Could you check a few things on this model? Use its own coordinates, in mm. Face numbers are marked on the shaded views. Coordinates: 2 decimals unless noted, no trailing zeros. Write each loop counter-clockwise with the first axis right and the second up, starting at its lowest first coordinate (ties: lowest second). Pieces come first, ordered by that corner, then holes. Notation, with made-up numbers: (52, 32) - (74, 32) arc R14 ccw to (74, 54) - close; hole circle Ø1 at (-24.75, 30.25). An arc over 180 degrees is marked (long way). Write item = value, one per line. Start each with the question number.
Autodesk Fusion 360 part; units mm, degrees
sketch "base Sketch" plane through (0, 0, 0) normal (0, 1, 0) x (1, 0, 0)
  line L0 (12.9, -8.5) -> (-12.9, -8.5)
  line L1 (-12.9, -8.5) -> (-12.9, 8.5)
  line L2 (-12.9, 8.5) -> (12.9, 8.5)
  line L3 (12.9, 8.5) -> (12.9, -8.5)
  line L4 (12.9, -8.5) -> (-12.9, 8.5) construction
  line L5 (-12.9, -8.5) -> (12.9, 8.5) construction
  circle A0 centre (5.625, 0) radius 2.775
  circle A1 centre (5.625, 0) radius 1.875
  circle A2 centre (-6.4, -0.0017) radius 2.0246 construction
  line L6 (-6.3962, -4.2517) -> (-2.7175, -2.1234)
  line L7 (-2.7175, -2.1234) -> (-2.7213, 2.1266)
  line L8 (-2.7213, 2.1266) -> (-6.4038, 4.2483)
  line L9 (-6.4038, 4.2483) -> (-10.0825, 2.12)
  line L10 (-10.0825, 2.12) -> (-10.0787, -2.13)
  line L11 (-10.0787, -2.13) -> (-6.3962, -4.2517)
  line L12 (-6.4027, 2.9781) -> (-8.9819, 1.4859)
  line L13 (-8.9819, 1.4859) -> (-8.9793, -1.4939)
  line L14 (-8.9793, -1.4939) -> (-6.3973, -2.9815)
  line L15 (-6.3973, -2.9815) -> (-3.8181, -1.4893)
  line L16 (-3.8181, -1.4893) -> (-3.8207, 1.4905)
  line L17 (-3.8207, 1.4905) -> (-6.4027, 2.9781)
  line L18 (-11.3, -6.9) -> (-11.3, 6.9)
  line L19 (-11.3, 6.9) -> (11.3, 6.9)
  line L20 (11.3, 6.9) -> (11.3, -6.9)
  line L21 (11.3, -6.9) -> (-11.3, -6.9)
  point P0 (-6.4, -0.0017)
  dimension "d1" = 25.8
  dimension "d2" = 17
  dimension "d3" = 5.55
  dimension "d4" = 7.275
  dimension "d5" = -0.9
  dimension "d6" = 6.5
  dimension "d7" = 4.25
  dimension "d8" = -1.1
  dimension "d15" = 1.6
extrude "Extrude1" add sketch "base Sketch" against normal blind 44 contours L0 L1 L2 L3 | A0 | A1 | L6 L7 L8 L9 L10 L11 | L12 L13 L14 L15 L16 L17 | L18 L19 L20 L21
extrude "Extrude2" add sketch "base Sketch" along normal blind 3.75 contours A0 | L6 L7 L8 L9 L10 L11
extrude "Extrude3" add sketch "base Sketch" along normal blind 1 contours L0 L1 L2 L3
fillet "Fillet1" radius 4 8 edges at (12.9, -21.5, 8.5) (-12.9, -21.5, 8.5) (-12.9, -21.5, -8.5) (12.9, -21.5, -8.5) (11.3, 0.5, 6.9) (-11.3, 0.5, 6.9) (-11.3, 0.5, -6.9) (11.3, 0.5, -6.9)
equation "d4 = 4.5 mm + d3 / 2"
equation "d7 = ( 8.5 / 2 ) * 1 mm"

Autodesk Fusion 360 part; units mm, degrees
sketch "Sketch1" plane through (0, 0, 0) normal (0, 1, 0) x (1, 0, 0)
  circle A0 centre (0, 0) radius 1.125
  circle A1 centre (0, 0) radius 3.5
  line L0 (0, 0) -> (13.95, 0) construction
  line L1 (0, 0) -> (-16.65, 0) construction
  line L2 (0, 0) -> (0, 6.5) construction
  line L3 (0, 0) -> (0, -6.5) construction
  circle A2 centre (0, 6.5) radius 1.9
  circle A3 centre (0, -6.5) radius 1.9
  circle A4 centre (13.95, 0) radius 1.95
  circle A5 centre (-16.65, 0) radius 1.95
  line L4 (14.0995, 1.9443) -> (1.9961, 2.875)
  line L5 (14.0995, -1.9443) -> (1.9961, -2.875)
  line L6 (-16.8396, 1.9408) -> (-1.9, 3.4)
  line L7 (1.9, 6.5) -> (1.9, 2.9394)
  line L8 (-1.9, 6.5) -> (-1.9, 3.4)
  line L9 (-1.9, -3.4) -> (-1.9, -6.5)
  line L10 (1.9, -2.9394) -> (1.9, -6.5)
  circle A6 centre (0, 0) radius 2.4
  circle A7 centre (8.35, 0) radius 0.45
  circle A8 centre (10.35, 0) radius 0.45
  circle A9 centre (12.35, 0) radius 0.45
  circle A10 centre (0, -6.15) radius 0.45
  circle A11 centre (0, -4.15) radius 0.45
  circle A12 centre (14.35, 0) radius 0.45
  circle A13 centre (6.35, 0) radius 0.45
  circle A14 centre (4.35, 0) radius 0.45
  line L11 (-16.8396, -1.9408) -> (-1.9, -3.4)
  circle A15 centre (0, 6.15) radius 0.45
  circle A16 centre (0, 4.15) radius 0.45
  circle A17 centre (-17.05, 0) radius 0.45
  circle A18 centre (-15.05, 0) radius 0.45
  circle A19 centre (-13.05, 0) radius 0.45
  circle A20 centre (-11.05, 0) radius 0.45
  circle A21 centre (-9.05, 0) radius 0.45
  circle A22 centre (-7.05, 0) radius 0.45
  circle A23 centre (-5.05, 0) radius 0.45
  circle A24 centre (0, 0) radius 2.3
  line L12 (1.9961, -2.875) -> (15.9, -2.875) construction
  line L13 (15.9, -2.875) -> (15.9, 0) construction
  line L14 (-1.9, -3.4) -> (-18.6, -3.4) construction
  line L15 (-18.6, -3.4) -> (-18.6, 0) construction
  line L16 (3.0895, -8.4) -> (-2.3757, -8.4) construction
  line L17 (0, -6.6) -> (0, -8.4) construction
  line L18 (-1.67, 8.4) -> (1.1298, 8.4) construction
  line L19 (0, 8.4) -> (0, 6.6) construction
  dimension "d1" = 3.8
  dimension "d2" = 3.9
  dimension "d3" = 3.8
  dimension "d4" = 3.9
  dimension "d6" = 16.65
  dimension "d9" = 7
  dimension "d10" = 2.25
  dimension "d11" = 2.875
  dimension "d12" = 2.875
  dimension "d22" = 0.9
  dimension "d23" = 0.9
  dimension "d24" = 0.9
  dimension "d25" = 0.9
  dimension "d29" = 0.35
  dimension "d30" = 0.9
  dimension "d33" = 0.9
  dimension "d34" = 2
  dimension "d35" = 2
  dimension "d36" = 2
  dimension "d41" = 0.4
  dimension "d42" = 2
  dimension "d43" = 2
  dimension "d44" = 0.9
  dimension "d45" = 0.9
  dimension "d48" = 3.4
  dimension "d49" = 3.4
  dimension "d51" = 3.1
  dimension "d52" = 3.1
  dimension "d55" = 0.9
  dimension "d56" = 0.9
  dimension "d57" = 0.9
  dimension "d58" = 0.9
  dimension "d59" = 0.9
  dimension "d60" = 0.9
  dimension "d61" = 0.9
  dimension "d62" = 0.9
  dimension "d63" = 0.9
  dimension "d64" = 0.4
  dimension "d65" = 2
  dimension "d66" = 2
  dimension "d67" = 2
  dimension "d68" = 2
  dimension "d69" = 2
  dimension "d70" = 2
  dimension "d72" = 4.6
  dimension "d73" = 1.1
  dimension "d76" = 4.8
  dimension "d81" = 13.9039
  dimension "d83" = 14
  dimension "d84" = 16.7
  dimension "d85" = 2
  dimension "d86" = 2
  dimension "d87" = 1.8
  dimension "d88" = 0.35
  dimension "d89" = 1.8
  dimension "d90" = 5
  dimension "d91" = 5.525
extrude "Extrude2" add sketch "Sketch1" along normal blind 4 contours A1 | A6 | A24
extrude "Extrude3" add sketch "Sketch1" along normal blind 1.5 contours A1 A4 L4 L5 A9 | A1 A2 A3 A5 L6 L7 L8 L9 L10 L11 A18 | A4 A9 | A2 | A4 A9 | A3 | A5 A18 | A5 A18 picked at (13.1485, 0.7143) picked at (11.9689, -0.0104) picked at (-15.8899, -0.7443) picked at (-14.6688, -0.0538)
extrude "Extrude4" cut sketch "Sketch1" along normal blind 1 contours A24
extrude "Extrude5" cut sketch "Sketch1" against normal blind 2.35 from surface at 4 contours A6 | A24
equation "d3 = d1"
equation "d6 = 18.6 mm - d4 / 2"
equation "d11 = ( 5.75 / 2 ) * 1 mm"
equation "d12 = d11"
equation "d22 = smallHoles"
equation "d23 = smallHoles"
equation "d24 = smallHoles"
equation "d25 = smallHoles"
equation "d29 = 1.8 mm - d3 / 2 + d25 / 2"
equation "d30 = smallHoles"
equation "d33 = smallHoles"
equation "d34 = 2.9 mm - d33"
equation "d35 = d34"
equation "d36 = d34"
equation "d41 = d2 / 2 - ( 1.1 mm + d33 / 2 )"
equation "d42 = d34"
equation "d43 = d34"
equation "d44 = smallHoles"
equation "d45 = smallHoles"
equation "d51 = 5 mm - d3 / 2"
equation "d52 = 5 mm - d1 / 2"
equation "d55 = smallHoles"
equation "d56 = smallHoles"
equation "d57 = smallHoles"
equation "d58 = smallHoles"
equation "d59 = smallHoles"
equation "d60 = smallHoles"
equation "d61 = smallHoles"
equation "d62 = smallHoles"
equation "d63 = smallHoles"
equation "d64 = d4 / 2 - ( 1.1 mm + d57 / 2 )"
equation "d65 = 2.9 mm - d57"
equation "d66 = d65"
equation "d67 = d65"
equation "d68 = d65"
equation "d69 = d65"
equation "d70 = d65"
equation "smallHoles = 0.9 mm"
equation "d85 = 2.9 mm - smallHoles"
equation "d86 = 2.9 mm - smallHoles"
equation "d88 = 1.8 mm - d1 / 2 + d56 / 2"
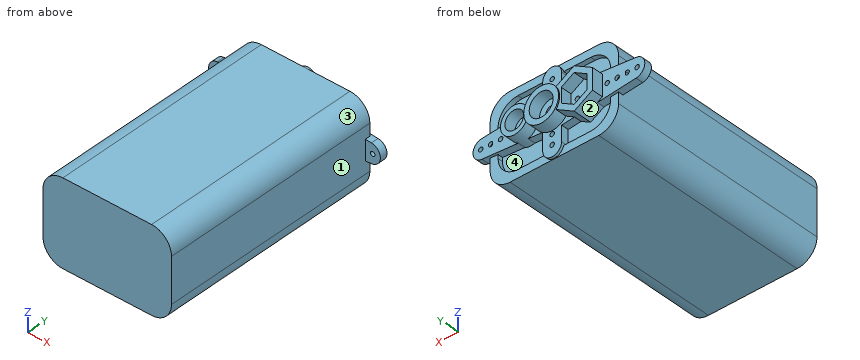
1) Thinking about a two-plate mould opening in Z: for the marked faces 1, 2, 3 and 4, which applies, +Z half, -Z half, draft (parallel to the pull), parting line (faces both ways), or undercut?
2) If I drill on probe 1 along Z at (x, y) = (0, 0.4); probe 2 along Y at (x, z) = (11, -7.5); probe 3 along X at (y, z) = (-0.5, 2), over which ranges is the centre line in solid material (lowest first)? Write a range as [from, to].
3) For P1, Ø5, axis at x = -16, z = -0.5, coming from the -Y side; P2, Ø1.9, axis at x = -0.5, z = 5, coming from the +Y side; P3, Ø0.5, axis at x = 8.5, z = 0, coming from the +Y side, each with a flat end and sliding along its axis, tell me the tip position at first contact or that it passes through.
4) Suppose I cut it at A-A on y = -5. Please give me the cut outline in (x, z), plus the area to 3 significant figures.
Reply:
q1.face_1 = draft
q1.face_2 = undercut
q1.face_3 = +Z half
q1.face_4 = undercut
q2.probe_1 = [-8.5, -6.6], [-5.7, -4.6], [-3.7, -2.3], [2.3, 3.7], [4.6, 5.7], [6.6, 8.5]
q2.probe_2 = [-44, 1]
q2.probe_3 = [-12.9, 12.9]
q3.P1 = 0
q3.P2 = 1.5
q3.P3 = 3.75
q4.outline = (-12.9, -4.5) arc R4 ccw to (-8.9, -8.5) - (8.9, -8.5) arc R4 ccw to (12.9, -4.5) - (12.9, 4.5) arc R4 ccw to (8.9, 8.5) - (-8.9, 8.5) arc R4 ccw to (-12.9, 4.5) - close
q4.area = 425 mm^2
